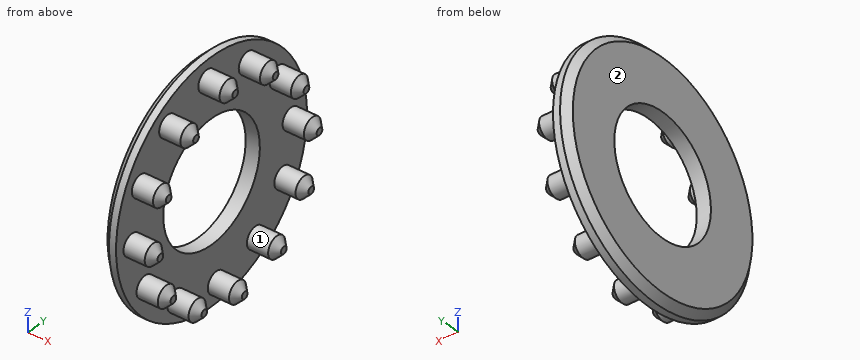
Autodesk Inventor part; units mm, degrees
ref_plane "YZ Plane" through (0, 0, 0) normal (1, 0, 0) x (0, 1, 0)
ref_plane "XZ Plane" through (0, 0, 0) normal (0, 1, 0) x (-1, 0, 0)
ref_plane "XY Plane" through (0, 0, 0) normal (0, 0, 1) x (1, 0, 0)
sketch "Skizze1" plane through (0, 0, 0) normal (0, 0, 1) x (1, 0, 0)
  point P0 (0, 0)
sketch "Skizze2" plane through (0, 0, 0) normal (1, 0, 0) x (0, 1, 0)
  circle A0 centre (0, 0) radius 8.4
  dimension "d0" = 16.8
extrude "Extrusion1" add sketch "Skizze2" along normal blind 1
sketch "Skizze3" plane through (1, 0, 0) normal (1, 0, 0) x (0, 0, -1)
  circle A0 centre (0, 0) radius 8.4
  circle A1 centre (-0.4149, 7) radius 0.75
  dimension "d3" = 1.5
  dimension "d4" = 7
extrude "Extrusion2" add sketch "Skizze3" along normal blind 2 contours A1
chamfer "Fase1" distance 0.5 angle 45 1 edges at (3, 7, 1.1649)
pattern_circular "Runde Anordnung1" count 12 over 360 about axis through (0, 0, 0) along (1, 0, 0) of "Extrusion2", "Fase1"
sketch "Skizze4" plane through (1, 0, 0) normal (1, 0, 0) x (0, 0, -1)
  circle A0 centre (0, 0) radius 8.4
  circle A1 centre (0, 0) radius 4.25
  dimension "d16" = 8.5
extrude "Extrusion3" cut sketch "Skizze4" against normal up to next contours A1
chamfer "Fase3" distance 0.5 angle 45 1 edges at (0, -8.4, 0)
properties part number "Servoscheibenflansch"
Source: CAD feature listing. Evaluate the final solid. Frame: model axes, mm. Face numbers are marked on the shaded views. Give positions to 0.01 mm unless a question says otherwise; leave off trailing zeros. Write each loop counter-clockwise with the first axis right and the second up, starting at its lowest first coordinate (ties: lowest second). Pieces come first, ordered by that corner, then holes. Notation, with made-up numbers: (-4.75, 45.25) -> (25.25, 45.25) arc R11 cw to (25.25, 51.25) -> close; hole circle Ø11 at (82, -32.75). An arc over 180 degrees is marked (long way). Return JSON: item names as keys, results as strings. Group by question number.
1. Section A-A, the plane x = 0.8. Output: boundary loops of the cut face in (y, z).
2. Pin query (flat end, axial travel): pin 1 Ø1.5 at (y, z) = (4.5, -1) entering from +X; pin 2 Ø6 at (y, z) = (1.5, 2.5) entering from -X. Return the tip coordinate at first contact, or that it passes through.
3. Material intervals for line 1 (Z direction, x = 1.45, y = -3.5); line 2 (X direction, y = 7.5, z = -0.5); line 3 (Y direction, x = 2.1, z = 3.25), sorted ascending. Write a range as from..to.
4. Mould query, pull axis Y, two halves, no side actions, for the marked faces 1 and 2. Classes: +Y half, -Y half, draft (parallel to the pull), parting line (faces both ways), or undercut.
Determined:
{
 "1": {"outline": "circle Ø16.8 at (0, 0); hole circle Ø8.5 at (0, 0)"},
 "2": {"pin 1": "stops at x = 1", "pin 2": "stops at x = 0"},
 "3": {"line 1": "z = -6.93..-5.61, 5.2..6.51", "line 2": "x = 0..1", "line 3": "y = -7.01..-5.53, 5.42..6.29"},
 "4": {"face 1": "undercut", "face 2": "draft"}
}
